The drawing under review shows one solid part. Ordinate dimensions are in mm from its lowest x, y, z. Coordinates: 2 decimals unless noted, no trailing zeros. Order: outer loops, then holes, each group sorted by start corner. A loop starts at its lowest first (then second) coordinate and runs counter-clockwise, first axis right, second up.
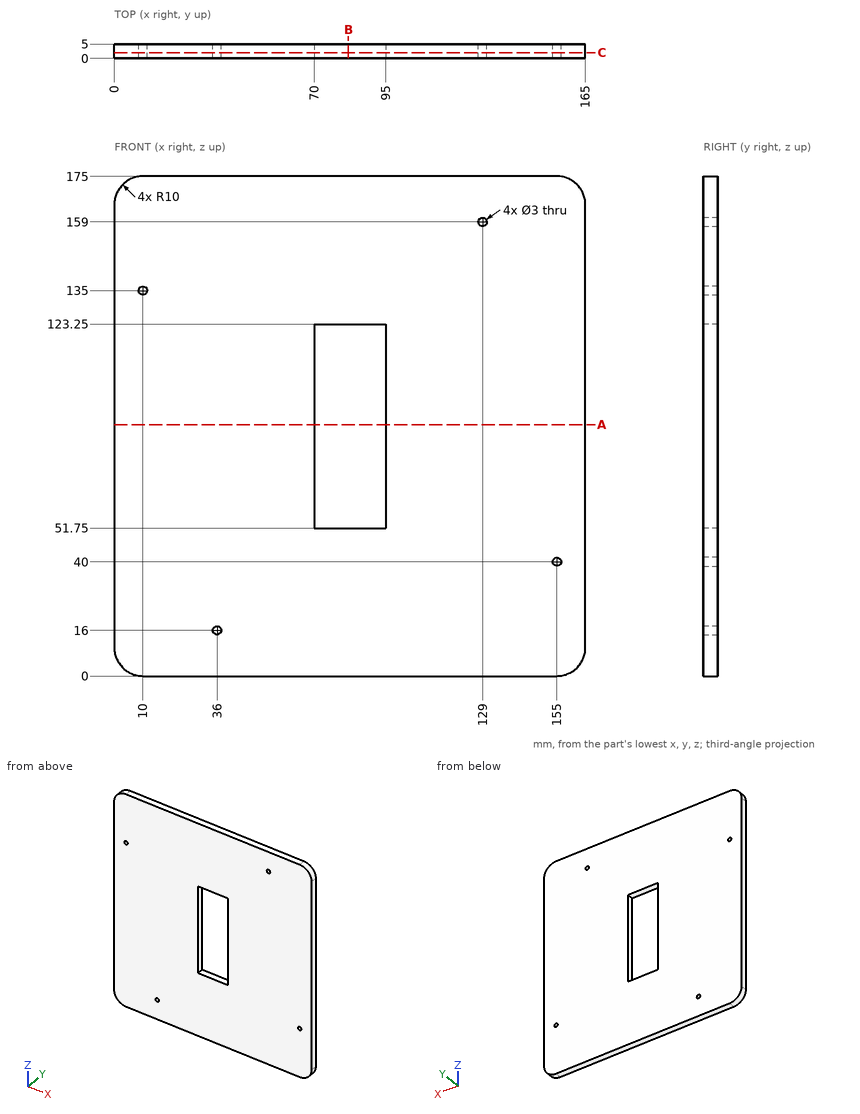
(1) Consider section B-B (x = 82). Give the boundary of the cut face in (y, z).
(2) Consider section A-A (z = 88). Give the boundary of the cut face in (x, y), then the cut area to 3 significant figures.
(3) Consider section C-C (y = 2). Give the boundary of the cut face in (x, z), then the cut area to 3 significant figures.
(4) Wall thickness on line 1 (X direction, y = 2.4, z = 52); line 2 (Z direction, x = 155, y = 1.15); line 3 (X direction, y = 3.35, z = 135): over which ranges is each line inside the solid? List them lowest first.
(5) Insertion check: pin 1 Ø2.5 at (x, z) = (155, 40) entering from -Y. The pin has a flat end and moves straight along its axis. Give the tip position at first contact, or say it passes through.
Findings:
1. outline: (0, 0) - (5, 0) - (5, 51.75) - (0, 51.75) - close; (0, 123.25) - (5, 123.25) - (5, 175) - (0, 175) - close
2. outline: (0, 0) - (70, 0) - (70, 5) - (0, 5) - close; (95, 0) - (165, 0) - (165, 5) - (95, 5) - close
2. area: 700 mm2
3. outline: (0, 10) arc R10 ccw to (10, 0) - (155, 0) arc R10 ccw to (165, 10) - (165, 165) arc R10 ccw to (155, 175) - (10, 175) arc R10 ccw to (0, 165) - close; hole circle Ø3 at (10, 135); hole circle Ø3 at (36, 16); hole (70, 51.75) - (95, 51.75) - (95, 123.25) - (70, 123.25) - close; hole circle Ø3 at (129, 159); hole circle Ø3 at (155, 40)
3. area: 27,000 mm2
4. line 1: x = 0 to 70, 95 to 165
4. line 2: z = 0 to 38.5, 41.5 to 175
4. line 3: x = 0 to 8.5, 11.5 to 165
5. pin 1: passes through
